Could you check a few things on this model? Use its own coordinates, in mm. Face numbers are marked on the shaded views. A direction names the side the tool comes from. Coordinates: 2 decimals unless noted, no trailing zeros. Order: outer loops, then holes, each group sorted by start corner. A loop starts at its lowest first (then second) coordinate and runs counter-clockwise, first axis right, second up. Notation, with made-up numbers: (-37, 75.5) - (9, 75.5) arc R11 ccw to (9, 89.5) - close; hole circle Ø9 at (-36.5, -36.5). An arc over 180 degrees is marked (long way). One line per item, written item: value.
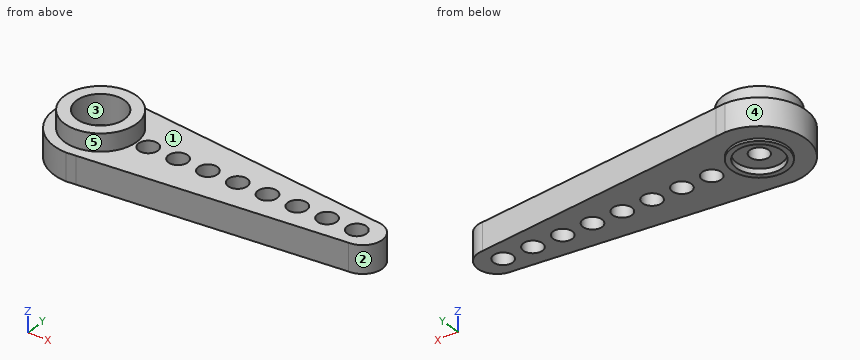
from build123d import *

# Parameters (mm, degrees)
EXTRUDE_1_DEPTH        = 4.58
SKETCH_2_R             = 6
EXTRUDE_2_DEPTH        = 2.9
SKETCH_3_R             = 4
CUT_EXTRUDE_1_DEPTH    = 4.935
SKETCH_6_R             = 4.65
EXTRUDE_3_DEPTH        = 0.4
SKETCH_7_R             = 3.8
CUT_EXTRUDE_4_DEPTH    = 0.9
SKETCH_4_R             = 1.575
CUT_EXTRUDE_2_DEPTH    = 3.945
SKETCH_5_R             = 1.6
CUT_EXTRUDE_3_DEPTH    = 8.48
PATTERN_LINEAR_1_COUNT = 8
PATTERN_LINEAR_1_PITCH = 5


with BuildPart() as part:
    # 草圖1 → 填料-伸長1 (new body)
    with BuildSketch(Plane.XY):
        with BuildLine():
            Line((1.568817891, 7.589552716), (0, 7.75))
            ThreePointArc((0, 7.75), (-7.75, 0), (0, -7.75))
            Line((0, -7.75), (1.568817891, -7.589552716))
            Line((1.568817891, -7.589552716), (44, -3.25))
            ThreePointArc((44, -3.25), (47.25, 0), (44, 3.25))
            Line((44, 3.25), (1.568817891, 7.589552716))
        make_face()
    extrude(amount=EXTRUDE_1_DEPTH)

    # 草圖2 → 填料-伸長2 (add)
    with BuildSketch(Plane.XY.offset(4.58)):
        Circle(SKETCH_2_R)
    extrude(amount=EXTRUDE_2_DEPTH)

    # 草圖3 → 除料-伸長1 (cut)
    with BuildSketch(Plane.XY.offset(7.48)):
        Circle(SKETCH_3_R)
    extrude(amount=-CUT_EXTRUDE_1_DEPTH, mode=Mode.SUBTRACT)

    # 草圖6 → 填料-伸長3 (add)
    with BuildSketch(Plane(origin=(0, 0, 0), x_dir=(-1, 0, 0), z_dir=(0, 0, -1))):
        Circle(SKETCH_6_R)
    extrude(amount=EXTRUDE_3_DEPTH)

    # 草圖7 → 除料-伸長4 (cut)
    with BuildSketch(Plane(origin=(0, 0, -0.4), x_dir=(-1, 0, 0), z_dir=(0, 0, -1))):
        Circle(SKETCH_7_R)
    extrude(amount=-CUT_EXTRUDE_4_DEPTH, mode=Mode.SUBTRACT)

    # 草圖4 → 除料-伸長2 (cut, through all)
    with BuildSketch(Plane.XY.offset(2.545)):
        Circle(SKETCH_4_R)
    extrude(amount=-CUT_EXTRUDE_2_DEPTH, mode=Mode.SUBTRACT)

    # 草圖5 → 除料-伸長3 (cut, through all)
    with BuildSketch(Plane(origin=(0, 0, 0), x_dir=(-1, 0, 0), z_dir=(0, 0, -1))):
        with Locations((-8, 0)):
            Circle(SKETCH_5_R)
    cut_extrude_3 = extrude(amount=-CUT_EXTRUDE_3_DEPTH, mode=Mode.SUBTRACT)

    # 直線複製排列1: 除料-伸長3 ×8
    with Locations(*[(i * PATTERN_LINEAR_1_PITCH, 0, 0) for i in range(1, PATTERN_LINEAR_1_COUNT)]):
        add(cut_extrude_3, mode=Mode.SUBTRACT)


solid = part.part
Item 1: I'm going to push flat-ended pins straight in: pin 1 Ø4 at (x, y) = (8, 0) entering from -Z; pin 2 Ø5 at (x, y) = (29, -2.5) entering from +Z; pin 3 Ø7 at (x, y) = (0, 0) entering from +Z (3 decimals). Where does each tip first touch, or does it pass through?
Conclusion:
pin 1: z = 0
pin 2: z = 4.58
pin 3: z = 2.545
Item 2: I want a section at B-B on x = 13. Please give me the cut outline in (y, z), then the cut area to 3 significant figures.
Conclusion:
outline: (-6.42, 0) - (-1.6, 0) - (-1.6, 4.58) - (-6.42, 4.58) - close; (1.6, 0) - (6.42, 0) - (6.42, 4.58) - (1.6, 4.58) - close
area: 44.2 mm²
Item 3: I want a section at A-A on z = 1.5. Give the number of separate pieces and of enclosed holes in the cut face, then the cut area to 3 significant figures.
Conclusion:
separate pieces: 1
enclosed holes: 9
area: 523 mm²
Item 4: I want a section at D-D on x = 28. Please give me the cut outline in (y, z).
Conclusion:
outline: (-4.89, 0) - (-1.6, 0) - (-1.6, 4.58) - (-4.89, 4.58) - close; (1.6, 0) - (4.89, 0) - (4.89, 4.58) - (1.6, 4.58) - close
Item 5: Thinking about a two-plate mould opening in X: for the marked faces 1, 2 and 3, which applies, pulls with the +X half, pulls with the -X half, needs draft (parallel to the pull), parting line crosses it, or undercut?
Conclusion:
face 1: needs draft
face 2: pulls with the +X half
face 3: undercut
Item 6: If I drill on probe 1 along Y at (x, z) = (0, 0.9) (3 decimals); probe 2 along Z at (x, y) = (24, 2); probe 3 along X at (y, z) = (-0.25, 5.5), over which ranges is the centre line in solid material (lowest first)?
Conclusion:
probe 1: -7.75 to -1.575, 1.575 to 7.75
probe 2: 0 to 4.58
probe 3: -5.99 to -3.99, 3.99 to 5.99
Item 7: For the marked faces 4 and 5, which set-ups out of +Z, -Z, +X, -X, +Y, -Y let a thin tool reach every point of the face, with its end or its side?
Conclusion:
face 4: +Z, -Z, -X
face 5: +Z
Item 8: I want a section at C-C on y = 5.5. Please give me the cut outline in (x, z).
Conclusion:
outline: (-5.46, 0) - (22, 0) - (22, 4.58) - (2.4, 4.58) - (2.4, 7.48) - (-2.4, 7.48) - (-2.4, 4.58) - (-5.46, 4.58) - close
